Check sheet for the modelled part. Datum: model origin and axes. Units: mm. A direction names the side the tool comes from. Round coordinates to 2 decimals unless told otherwise and drop trailing zeros. Write each loop counter-clockwise with the first axis right and the second up, starting at its lowest first coordinate (ties: lowest second). Pieces come first, ordered by that corner, then holes.
Autodesk Inventor part; units mm, degrees
ref_plane "Mezzeria" through (0, -5, 7.5) normal (0, -1, 0) x (1, 0, 0)
ref_plane "YZ Plane" through (0, 0, 0) normal (1, 0, 0) x (0, 1, 0)
ref_plane "XZ Plane" through (0, 0, 0) normal (0, 1, 0) x (-1, 0, 0)
sketch "Schizzo1" plane through (0, 0, 0) normal (0, 0, 1) x (1, 0, 0)
  line L0 (-12.5, 60) -> (-12.5, 0)
  line L1 (-12.5, 0) -> (12.5, 0)
  line L2 (12.5, 0) -> (12.5, 60)
  line L3 (12.5, 60) -> (7.5, 60)
  line L4 (7.5, 60) -> (7.5, 5)
  line L5 (7.5, 5) -> (-7.5, 5)
  line L6 (-7.5, 5) -> (-7.5, 60)
  line L7 (-7.5, 60) -> (-12.5, 60)
  point P0 (0, 0)
  point P1 (0, 5)
  point P2 (0, 0)
  dimension "d0" = 25
  dimension "d1" = 15
  dimension "d2" = 5
  dimension "d3" = 60
extrude "Estrusione1" add sketch "Schizzo1" along normal blind 15
sketch "Schizzo2" plane through (0, 0, 0) normal (1, 0, 0) x (0, 1, 0)
  line L0 (5, 0) -> (60, 0)
  line L1 (60, 0) -> (60, 15)
  line L2 (5, 15) -> (60, 15)
  line L3 (5, 0) -> (5, 15)
  circle A0 centre (50, 7.5) radius 5
  point P0 (0, 0)
  point P1 (60, 7.5)
  point P2 (32.5, 0)
  dimension "d6" = 10
  dimension "d28" = 10
extrude "Estrusione2" cut sketch "Schizzo2" along normal through all both and the other way through all contours A0
fillet "Raccordo1" radius 2 6 edges at (-10, 60, 15) (-10, 60, 0) (10, 60, 15) (10, 60, 0) (12.5, 0, 7.5) (-12.5, 0, 7.5)
sketch "Schizzo3" plane through (-10.5, 0, 0) normal (0, -1, 0) x (1, 0, 0)
  line L0 (0, 0) -> (0, 15)
  line L1 (0, 0) -> (21, 0)
  line L2 (21, 15) -> (21, 0)
  line L3 (0, 15) -> (21, 15)
  circle A0 centre (10.5, 7.5) radius 6
  point P0 (10.5, 0)
  point P1 (21, 7.5)
  point P2 (10.5, 0)
  dimension "d13" = 12
extrude "Estrusione3" add sketch "Schizzo3" along normal blind 10 contours A0
ref_plane "Mezzeria" through (0, -5, 7.5) normal (0, -1, 0) x (1, 0, 0)
mirror "Specchio2" about plane through (0, -5, 7.5) normal (0, -1, 0) of "Estrusione1"
mirror "Specchio3" about plane through (0, -5, 7.5) normal (0, -1, 0) of "Estrusione2", "Raccordo1"
chamfer "Smusso1" distance 0.5 angle 45 8 edges at (-7.5, 45, 7.5) (7.5, 45, 7.5) (-12.5, 45, 7.5) (12.5, 45, 7.5) (12.5, -55, 7.5) (7.5, -55, 7.5) (-7.5, -55, 7.5) (-12.5, -55, 7.5)
properties part number "Forcella movimento lama" material "Acciaio inossidabile"
1. Sectioned sample at C-C, the plane z = 7.5. Give the number of separate pieces and of enclosed holes in the cut face, plus the area to 3 significant figures.
2. Scan lines: line 1 along Y through (x, z) = (-4, 13); line 2 along X through (y, z) = (-38, 3.25); line 3 along Z through (x, y) = (11.1, -60). Record each from-to range of solid material in increasing order.
3. Set-up check for faces 5 (the flat face through (0, 0, 14)), 6 (the cylindrical face through (11.9, 0.57, 7.6)), 7 (the flat face through (7.5, -42, 7)): record each of +Z, -Z, +X, -X, +Y, -Y from which the full face is reachable in a straight line by a thin tool's end or side.
4. Release check for a two-part mould opening along Y. For faces 1 (the cylindrical face through (-4.42, -4.93, 3.44)), 2 (the flat face through (-7.5, 32, 7)), 3 (the cylindrical face through (9.96, -69.4, 0.57)), 4 (the cylindrical face through (-9.972, 46.315, 10.879)) record: released by +Y, released by -Y, zero draft, split by the parting line, or undercut.
5. Sectioned sample at B-B, the plane y = -60. Enter the section's corners in (x, z).
6. Sectioned sample at D-D, the plane x = 0. Enter the section's corners in (y, z).
7. Go/stop test with flat-tipped pins: pin 1 (4.5 mm diameter, centred on x = -3, z = 6, fed in from -Y); pin 2 (4.5 mm diameter, centred on x = 2.5, z = 7, fed in from +Y). Record where each tip stops, or that it passes through.
8. Sectioned sample at A-A, the plane y = -44.5. Enter the section's corners in (x, z), plus the area to 3 significant figures.
Computed values:
1. separate pieces: 5
1. enclosed holes: 0
1. area: 1,260 mm2
2. line 1: y = -15 to -10, 0 to 5
2. line 2: x = -12.5 to -7.5, 7.5 to 12.5
2. line 3: z = 0 to 2.5, 12.5 to 15
3. face 5: none
3. face 6: +Z, -Z, +X
3. face 7: +Z, -Z, -Y
4. face 1: undercut
4. face 2: zero draft
4. face 3: released by -Y
4. face 4: undercut
5. outline: (-12.5, 0) - (-7.5, 0) - (-7.5, 2) - (-8, 2.5) - (-12, 2.5) - (-12.5, 2) - close; (-12.5, 13) - (-12, 12.5) - (-8, 12.5) - (-7.5, 13) - (-7.5, 15) - (-12.5, 15) - close; (7.5, 0) - (12.5, 0) - (12.5, 2) - (12, 2.5) - (8, 2.5) - (7.5, 2) - close; (7.5, 13) - (8, 12.5) - (12, 12.5) - (12.5, 13) - (12.5, 15) - (7.5, 15) - close
6. outline: (-15, 0) - (-10, 0) - (-10, 1.5) - (0, 1.5) - (0, 0) - (5, 0) - (5, 15) - (0, 15) - (0, 13.5) - (-10, 13.5) - (-10, 15) - (-15, 15) - close
7. pin 1: stops at y = -15
7. pin 2: stops at y = 5
8. outline: (-12.5, 0) - (-7.5, 0) - (-7.5, 15) - (-12.5, 15) - close; (7.5, 0) - (12.5, 0) - (12.5, 15) - (7.5, 15) - close
8. area: 150 mm2
